Input: part model. Units: mm. Frame: model coordinates. Face numbers are marked on the shaded views. A direction names the side the tool comes from. Round coordinates to 2 decimals unless told otherwise and drop trailing zeros. Loops run counter-clockwise (first coordinate to the right, second up) from the corner with the lowest first, then second, coordinate; pieces in that order, holes last. Notation, with made-up numbers: (70.5, -35.5) -> (98.5, -35.5) arc R8 ccw to (98.5, -31.5) -> close; hole circle Ø1 at (69, 19). An arc over 180 degrees is marked (long way). Answer as a JSON object with one key per item and string values. Group by question number.
Item 1: Section query C-C on x = -18.5. Return loops of the section in (y, z).
Item 2: Section query B-B on z = -57. Return loops of the section in (x, y).
Item 3: Pin query (flat end, axial travel): pin 1 (7 mm diameter, centred on y = 31.5, z = -35.5, fed in from -X); pin 2 (6 mm diameter, centred on x = -23, y = 9.5, fed in from -Z); pin 3 (9 mm diameter, centred on y = 38.5, z = -48, fed in from +X). Return the tip coordinate at first contact, or that it passes through.
Item 4: Set-up query: the marked faces 4, 5, 6 and 7. Return all of +Z, -Z, +X, -X, +Y, -Y with unobstructed straight access to the full face (end or side cutting, diameter ignored); none if empty.
Item 5: Section query D-D on z = -80. Return loops of the section in (x, y), and give its area (3 significant figures).
Item 6: Section query A-A on y = 10. Return loops of the section in (x, z).
Item 7: Draft query along Z for the marked faces 1, 2 and 3. Return one class per face: released by +Z, released by -Z, zero draft, split by the parting line, or undercut.
Item 8: Material intervals for line 1 (Y direction, x = -5, z = -80); line 2 (Z direction, x = -3.5, y = 10); line 3 (X direction, y = 51.5, z = -72), sorted ascending. Write a range as [from, to].
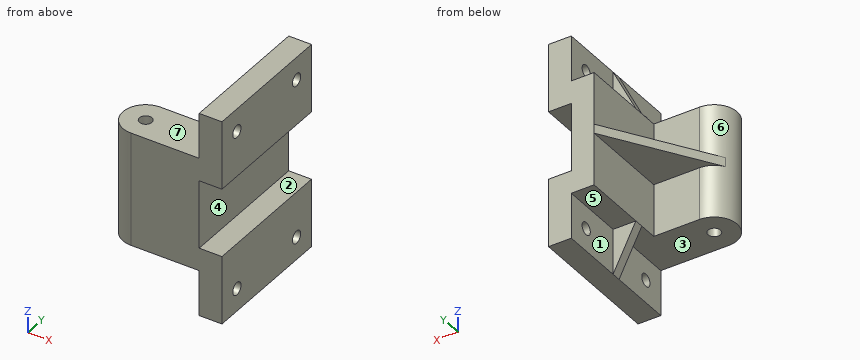
Autodesk Inventor part; units mm, degrees
ref_plane "Work Plane1" through (-20, 20, -47) normal (0, 0, -1) x (-1, 0, 0)
ref_plane "YZ Plane" through (0, 0, 0) normal (1, 0, 0) x (0, 1, 0)
ref_plane "XZ Plane" through (0, 0, 0) normal (0, 1, 0) x (-1, 0, 0)
sketch "Sketch1" plane through (0, 0, 0) normal (0, 1, 0) x (-1, 0, 0)
  line L0 (0, 0) -> (10, 0)
  line L1 (0, 0) -> (0, -30)
  line L2 (0, -30) -> (10, -30)
  line L3 (10, -30) -> (10, -60)
  line L4 (10, -60) -> (0, -60)
  line L5 (0, -60) -> (0, -90)
  line L6 (0, -90) -> (10, -90)
  line L7 (10, -90) -> (10, -70)
  line L8 (10, -70) -> (20, -70)
  line L9 (20, -70) -> (20, -20)
  line L10 (20, -20) -> (10, -20)
  line L11 (10, -20) -> (10, 0)
  dimension "d0" = 10
  dimension "d1" = 30
  dimension "d2" = 10
  dimension "d3" = 30
  dimension "d4" = 10
  dimension "d5" = 30
  dimension "d6" = 10
  dimension "d7" = 20
  dimension "d8" = 10
  dimension "d9" = 50
extrude "Extrusion1" add sketch "Sketch1" along normal blind 60
sketch "Sketch2" plane through (-10, 0, -90) normal (-1, 0, 0) x (0, 0, 1)
  line L0 (30, 60) -> (0, 60)
  line L1 (0, 60) -> (0, 32)
  line L2 (0, 0) -> (0, 60)
  line L3 (0, 32) -> (20, 32)
  line L4 (20, 32) -> (20, 28)
  line L5 (20, 28) -> (0, 28)
  line L6 (0, 28) -> (0, 32)
  line L7 (60, 60) -> (30, 60)
  line L8 (45, 60) -> (45, 0)
  line L9 (60, 0) -> (30, 0)
  line L10 (90, 0) -> (90, 60)
  line L11 (90, 32) -> (70, 32)
  line L12 (70, 32) -> (70, 28)
  line L13 (70, 28) -> (90, 28)
  line L14 (90, 28) -> (90, 32)
  dimension "d12" = 28
  dimension "d13" = 20
  dimension "d14" = 4
extrude "Extrusion2" add sketch "Sketch2" along normal blind 10
sketch "Sketch3" plane through (-10, 32, -70) normal (0, 1, 0) x (1, 0, 0)
  line L0 (-10, 0) -> (-10, -50)
  line L1 (10, 20) -> (0, 20)
  line L2 (-10, 0) -> (0, 20)
  line L3 (0, 20) -> (-10, 20)
  line L4 (-10, 0) -> (-10, 20)
  line L5 (-10, 20) -> (-10, 0)
  line L6 (-10, -50) -> (0, -50)
  line L7 (0, -70) -> (10, -70)
  line L8 (-10, -50) -> (0, -70)
  line L9 (0, -70) -> (-10, -70)
  line L10 (-10, -70) -> (-10, -50)
extrude "Extrusion3" cut sketch "Sketch3" against normal blind 10
sketch "Sketch4" plane through (-10, 0, -70) normal (0, 0, -1) x (-1, 0, 0)
  line L0 (0, 32) -> (0, 60)
  line L1 (0, 60) -> (0, 10)
  line L2 (0, 10) -> (30, 10) construction
  circle A0 centre (30, 10) radius 2.75
  arc A1 (30, 0) -> (30, 20) centre (30, 10) ccw
  line L3 (10, 0) -> (0, 0)
  line L4 (0, 0) -> (30, 0)
  line L5 (0, 0) -> (0, 28)
  line L6 (0, 0) -> (0, 20)
  line L7 (0, 20) -> (30, 20)
  line L8 (10, 0) -> (10, 28)
  line L9 (10, 20) -> (10, 0)
  point P0 (-10, 0)
  dimension "d19" = 50
  dimension "d20" = 30
  dimension "d21" = 5.5
  dimension "d22" = 20
extrude "Extrusion4" add sketch "Sketch4" against normal blind 50 contours L7 A1 L4 L8
ref_plane "Work Plane1" through (-20, 20, -47) normal (0, 0, -1) x (-1, 0, 0)
sketch "Sketch6" plane through (-20, 20, -47) normal (0, 0, -1) x (-1, 0, 0)
  line L0 (0, 40) -> (-10, 40)
  line L1 (0, 40) -> (28.4336, -4.6265)
  arc A0 (20, -20) -> (20, 0) centre (20, -10) ccw
  arc A1 (20, -20) -> (20, 0) centre (20, -10) ccw
  line L2 (28.4336, -4.6265) -> (-1.843, -4.6265)
  line L3 (-20, -20) -> (-20, 40)
  line L4 (-1.843, -4.6265) -> (-1.843, 40)
extrude "Extrusion6" add sketch "Sketch6" against normal blind 4
sketch "Sketch7" plane through (-10, 60, -90) normal (-1, 0, 0) x (0, 0, 1)
  line L0 (90, -28) -> (90, 0)
  line L1 (70, 0) -> (90, 0)
  line L2 (70, -60) -> (90, -60)
  line L3 (90, -60) -> (90, -32)
  line L4 (0, -60) -> (0, -32)
  line L5 (0, -60) -> (20, -60)
  line L6 (0, -28) -> (0, 0)
  line L7 (0, 0) -> (20, 0)
  point P0 (10, -10)
  point P1 (10, -50)
  point P2 (80, -50)
  point P3 (80, -10)
  dimension "d39" = 10
  dimension "d40" = 10
  dimension "d41" = 10
  dimension "d42" = 10
  dimension "d43" = 10
  dimension "d44" = 10
  dimension "d45" = 10
  dimension "d46" = 10
hole "Hole1" at (-10, 50, -80) at (-10, 10, -80) at (-10, 10, -10) at (-10, 50, -10) direction (1, 0, 0) diameter 5.5 end through all
properties part number "MMAE 232 Assignment 1d-Nicholas Skiba" material "Aluminum 6061"
Solved:
{
 "1": {"outline": "(0, -70) -> (28, -70) -> (28, -73) -> (32, -73) -> (32, -70) -> (60, -70) -> (60, -20) -> (32, -20) -> (32, -17) -> (28, -17) -> (28, -20) -> (0, -20) -> close"},
 "2": {"outline": "(-40, 0) -> (-10, 0) -> (-10, 60) -> (-20, 60) -> (-20, 20) -> (-40, 20) arc R10 ccw to start; hole circle Ø5.5 at (-40, 10)"},
 "3": {"pin 1": "x = -20", "pin 2": "z = -70", "pin 3": "x = -10"},
 "4": {"face 4": "+X, +Y, -Y", "face 5": "-Z, -X, +Y", "face 6": "-X", "face 7": "+Z, -X, -Y"},
 "5": {"outline": "(-15, 28) -> (-10, 28) -> (-10, 12.75) -> (0, 12.75) -> (0, 47.25) -> (-10, 47.25) -> (-10, 32) -> (-15, 32) -> close; (-10, 0) -> (0, 0) -> (0, 7.25) -> (-10, 7.25) -> close; (-10, 52.75) -> (0, 52.75) -> (0, 60) -> (-10, 60) -> close", "area": "510 mm²"},
 "6": {"outline": "(-50, -70) -> (-42.75, -70) -> (-42.75, -20) -> (-50, -20) -> close; (-37.25, -70) -> (-10, -70) -> (-10, -77.25) -> (0, -77.25) -> (0, -60) -> (-10, -60) -> (-10, -30) -> (0, -30) -> (0, -12.75) -> (-10, -12.75) -> (-10, -20) -> (-37.25, -20) -> close; (-10, -90) -> (0, -90) -> (0, -82.75) -> (-10, -82.75) -> close; (-10, -7.25) -> (0, -7.25) -> (0, 0) -> (-10, 0) -> close"},
 "7": {"face 1": "zero draft", "face 2": "undercut", "face 3": "released by -Z"},
 "8": {"line 1": "[0, 7.25], [12.75, 47.25], [52.75, 60]", "line 2": "[-90, -82.75], [-77.25, -60], [-30, -12.75], [-7.25, 0]", "line 3": "[-10, 0]"}
}
